```python
from build123d import *

# Parameters (mm, degrees)
SKETCH_1_R               = 21
EXTRUDE_1_DEPTH          = 4
EXTRUDE_2_DEPTH          = 4
PATTERN_CIRCULAR_1_COUNT = 8
CHAMFER_1_SIZE           = 0.5


with BuildPart() as part:
    # 草图1 → 凸台-拉伸1 (new body)
    with BuildSketch(Plane(origin=(0, 0, 0), x_dir=(1, 0, 0), z_dir=(0, 1, 0))):
        Circle(SKETCH_1_R)
    extrude(amount=EXTRUDE_1_DEPTH)

    # 草图2 → 凸台-拉伸2 (add)
    with BuildSketch(Plane(origin=(0, 4, 0), x_dir=(1, 0, 0), z_dir=(0, 1, 0))):
        with BuildLine():
            Line((-22.299103121, 3), (22.299103121, 3))
            ThreePointArc((22.299103121, 3), (22.5, 0), (22.299103121, -3))
            Line((22.299103121, -3), (-22.299103121, -3))
            ThreePointArc((-22.299103121, -3), (-22.5, 0), (-22.299103121, 3))
        make_face()
    extrude_2 = extrude(amount=-EXTRUDE_2_DEPTH)

    # 阵列(圆周)1: 凸台-拉伸2 ×8 about axis
    pattern_circular_1_axis = Axis((0, 0, 0), (0, 1, 0))
    for i in range(1, PATTERN_CIRCULAR_1_COUNT):
        add(extrude_2.rotate(pattern_circular_1_axis, i * 360 / PATTERN_CIRCULAR_1_COUNT))

    # 倒角1
    chamfer_1_edges = [part.edges().sort_by_distance(p)[0] for p in [
        (22.5, 4, 0),
        (-22.5, 4, 0),
        (15.909902577, 4, -15.909902577),
        (0, 4, -22.5),
        (-15.909902577, 4, -15.909902577),
        (15.909902577, 4, 15.909902577),
        (-15.909902577, 4, 15.909902577),
        (0, 4, 22.5),
    ]]
    chamfer(chamfer_1_edges, length=CHAMFER_1_SIZE)


solid = part.part
```
Work out the finished part from the listing and answer in its coordinate system (mm). A direction names the side the tool comes from. Give positions to 0.01 mm unless a question says otherwise; leave off trailing zeros. Order: outer loops, then holes, each group sorted by start corner. A loop starts at its lowest first (then second) coordinate and runs counter-clockwise, first axis right, second up. Notation, with made-up numbers: (17, 36) - (71, 36) arc R15 cw to (71, 41) - close; hole circle Ø5 at (54, 69.5). An arc over 180 degrees is marked (long way). One line per item, written item: value. Start each with the question number.
1. Consider line 1 (X direction, y = 3.55, z = 11); line 2 (Z direction, x = -17.5, y = 1.65); line 3 (X direction, y = 3.2, z = -2). Determine where each line is inside the solid, lowest interval first.
2. Which of the six approach directions +Z, -Z, +X, -X, +Y, -Y give full straight-line access (tool end or side, diameter ignored) to faces 1 (the face through (17.36, 2.03, -13.12)), 2 (the face through (-13.104, 2.028, 17.346)), 3 (the face through (-19.43, 1.97, 7.97)), 4 (the face through (22, 2, 3))?
3. Section B-B, the plane z = -19 is taken. Write down the section's boundary in (x, y).
4. Each of these flat-tipped pins is pushed along its axis until it touches: pin 1 Ø1.2 at (x, y) = (-22, 1.5) entering from -Z; pin 2 Ø10 at (x, z) = (-11, -7) entering from -Y; pin 3 Ø0.5 at (y, z) = (1.5, -21.5) entering from +X; pin 4 Ø0.5 at (y, z) = (2, 22) entering from -X. Where does it stop, or does it pass through?
5. Section C-C, the plane z = -11 is taken. Write down the section's boundary in (x, y), then the cut area to 3 significant figures.
6. For a pull along X with two mould halves and no side action, classify faces 5 (the face through (-15.726, 3.802, -15.666)), 6 (the face through (13.104, 2.028, -17.346)), 7 (the face through (15.726, 3.802, 15.666)) as released by +X, released by -X, zero draft, split by the parting line, or undercut.
Filled sheet:
1. line 1: -17.89 to 17.89
1. line 2: -14.14 to -13.26, -11.61 to 11.61, 13.26 to 14.14
1. line 3: -22.41 to 22.41
2. face 1: +X, +Y, -Y
2. face 2: +Z, +Y, -Y
2. face 3: -X, +Y, -Y
2. face 4: +Z, +X, +Y, -Y
3. outline: (-8.94, 0) - (8.94, 0) - (8.94, 4) - (-8.94, 4) - close
4. pin 1: z = -3
4. pin 2: y = 0
4. pin 3: x = 3
4. pin 4: x = -3
5. outline: (-17.89, 0) - (17.89, 0) - (17.89, 4) - (-17.89, 4) - close
5. area: 143 mm²
6. face 5: released by -X
6. face 6: undercut
6. face 7: released by +X
